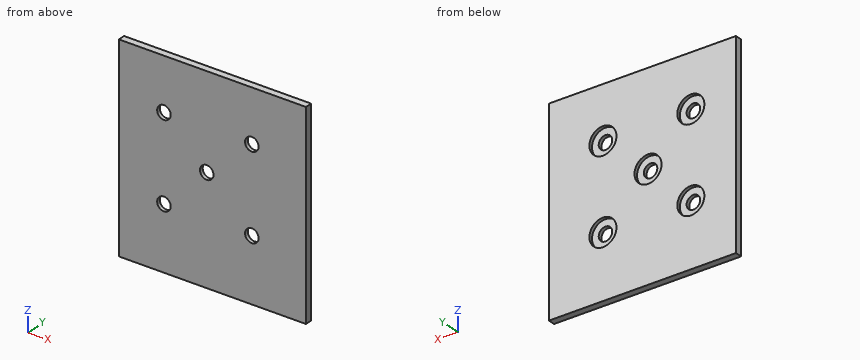
Autodesk Inventor part; units mm, degrees
ref_plane "YZ Plane" through (0, 0, 0) normal (1, 0, 0) x (0, 1, 0)
ref_plane "XZ Plane" through (0, 0, 0) normal (0, 1, 0) x (-1, 0, 0)
ref_plane "XY Plane" through (0, 0, 0) normal (0, 0, 1) x (1, 0, 0)
sketch "草圖1" plane through (0, 0, 0) normal (0, 1, 0) x (-1, 0, 0)
  line L0 (0, 0) -> (83, 0)
  line L1 (83, 0) -> (83, -87.8)
  line L2 (83, -87.8) -> (0, -87.8)
  line L3 (0, -87.8) -> (0, 0)
  dimension "d0" = 87.8
  dimension "d1" = 83
extrude "擠出1" add sketch "草圖1" along normal blind 3.1
sketch "草圖2" plane through (0, 3.1, 0) normal (0, 1, 0) x (1, 0, 0)
  line L0 (-24, -18.3432) -> (-24, 108.3328)
  line L1 (-63, -18.3432) -> (-63, 117.1807)
  line L2 (-93.8741, 60) -> (24.8173, 60)
  line L3 (19.8538, 23) -> (-101.6429, 23)
  line L4 (-44, -5.6109) -> (-44, 94.0899)
  line L5 (-89.7738, 41) -> (11.6533, 41)
  line L6 (-83, 0) -> (0, 0)
  line L7 (0, 0) -> (0, 87.8)
  circle A0 centre (-63, 23) radius 6
  circle A1 centre (-24, 23) radius 6
  circle A2 centre (-24, 60) radius 6
  circle A3 centre (-63, 60) radius 6
  circle A4 centre (-44, 41) radius 6
  dimension "d4" = 23
  dimension "d5" = 37
  dimension "d6" = 24
  dimension "d7" = 44
  dimension "d8" = 39
  dimension "d9" = 41
  dimension "d10" = 12
  dimension "d11" = 12
  dimension "d12" = 12
  dimension "d13" = 12
  dimension "d14" = 12
hole "孔1" at (-24, 3.1, -23) at (-63, 3.1, -23) at (-63, 3.1, -60) at (-24, 3.1, -60) direction (0, -1, 0) diameter 6 end through all
sketch "草圖4" plane through (0, 3.1, 0) normal (0, 1, 0) x (1, 0, 0)
  point P0 (0, 0)
sketch "草圖5" plane through (0, 3.1, 0) normal (0, 1, 0) x (1, 0, 0)
  circle A0 centre (-24, 23) radius 3
  circle A1 centre (-24, 23) radius 6
  point P0 (0, 0)
  dimension "d40" = 12
extrude "擠出2" cut sketch "草圖5" against normal blind 1.5
pattern_linear "矩形陣列2" count 2 spacing 39 along (-1, 0, 0) of "擠出2"
sketch "草圖6" plane through (0, 3.1, 0) normal (0, 1, 0) x (1, 0, 0)
  circle A0 centre (-63, 60) radius 3
  circle A1 centre (-63, 60) radius 6
  circle A2 centre (-24, 60) radius 3
  circle A3 centre (-24, 60) radius 6
  point P0 (0, 0)
  dimension "d46" = 12
  dimension "d47" = 12
extrude "擠出3" cut sketch "草圖6" against normal blind 1.5
sketch "草圖7" plane through (0, 3.1, 0) normal (0, 1, 0) x (1, 0, 0)
  circle A0 centre (-44, 41) radius 3
  line L0 (-83, 0) -> (0, 0)
  line L1 (0, 0) -> (0, 87.8)
  dimension "d50" = 6
  dimension "d51" = 41
  dimension "d52" = 44
extrude "擠出4" cut sketch "草圖7" against normal blind 5
sketch "草圖8" plane through (0, 3.1, 0) normal (0, 1, 0) x (1, 0, 0)
  circle A0 centre (-44, 41) radius 3
  circle A1 centre (-44, 41) radius 6
  point P0 (0, 0)
  dimension "d55" = 12
extrude "擠出5" cut sketch "草圖8" against normal blind 1.5
properties part number "底板" material "鋁合金 6061"
Can you work these out from the model? Positions are in its coordinate system, mm. Coordinates: 2 decimals unless noted, no trailing zeros. Order: outer loops, then holes, each group sorted by start corner. A loop starts at its lowest first (then second) coordinate and runs counter-clockwise, first axis right, second up. Notation, with made-up numbers: M 12,70.25 L 37,70.25 A35 cw 37,103.25 Z; hole C 8.25,29.25 d10. An arc over 180 degrees is marked long. Answer as CSV lines item,"result".
(1) Suppose I cut it at B-B on x = -44. Please give me the cut outline in (y, z).
Geometry check:
outline,"M 0,-87.8 L 3.1,-87.8 L 3.1,-47 L 1.6,-47 L 1.6,-44 L 0,-44 Z; M 0,-38 L 1.6,-38 L 1.6,-35 L 3.1,-35 L 3.1,0 L 0,0 Z"
(2) Suppose I cut it at D-D on z = -41. Please give me the cut outline in (x, y).
Geometry check:
outline,"M -83,0 L -47,0 L -47,1.6 L -50,1.6 L -50,3.1 L -83,3.1 Z; M -41,0 L 0,0 L 0,3.1 L -38,3.1 L -38,1.6 L -41,1.6 Z"
(3) I'm going to push flat-ended pins straight in: pin 1 (3.5 mm diameter, centred on x = -25, z = -58.5, fed in from +Y); pin 2 (5.5 mm diameter, centred on x = -63, z = -60, fed in from +Y). Where does each tip first touch, or does it pass through?
Geometry check:
pin 1,"y = 1.6"
pin 2,"through"
(4) Suppose I cut it at C-C on x = -63. Please give me the cut outline in (y, z).
Geometry check:
outline,"M 0,-87.8 L 3.1,-87.8 L 3.1,-66 L 1.6,-66 L 1.6,-63 L 0,-63 Z; M 0,-57 L 1.6,-57 L 1.6,-54 L 3.1,-54 L 3.1,-29 L 1.6,-29 L 1.6,-26 L 0,-26 Z; M 0,-20 L 1.6,-20 L 1.6,-17 L 3.1,-17 L 3.1,0 L 0,0 Z"
(5) Suppose I cut it at A-A on z = -23. Please give me the cut outline in (x, y).
Geometry check:
outline,"M -83,0 L -66,0 L -66,1.6 L -69,1.6 L -69,3.1 L -83,3.1 Z; M -60,0 L -27,0 L -27,1.6 L -30,1.6 L -30,3.1 L -57,3.1 L -57,1.6 L -60,1.6 Z; M -21,0 L 0,0 L 0,3.1 L -18,3.1 L -18,1.6 L -21,1.6 Z"
(6) Please list where these lines run through material, in increasing order: L1, parallel to X at y = 2.7, z = -60; L2, parallel to X at y = 1.25, z = -23; L3, parallel to Z at x = -63, y = 2.55.
Geometry check:
L1,"-83 to -69, -57 to -30, -18 to 0"
L2,"-83 to -66, -60 to -27, -21 to 0"
L3,"-87.8 to -66, -54 to -29, -17 to 0"
